Check sheet for the modelled part. Datum: model origin and axes. Units: mm. A direction names the side the tool comes from. Give positions to 0.01 mm unless a question says otherwise; leave off trailing zeros. Loops run counter-clockwise (first coordinate to the right, second up) from the corner with the lowest first, then second, coordinate; pieces in that order, holes last.
```python
from build123d import *

# Parameters (mm, degrees)
F0_W      = 127
F0_H      = 127
F1_DEPTH  = 7.62
F2_W      = 111.76
F2_H      = 7.62
F3_DEPTH  = 76.2
F4_W      = 25.4
F4_H      = 50.8
F5_DEPTH  = 7.62
F6_W      = 31.75
F6_H      = 19.05
F7_DEPTH  = 7.62
F8_W      = 38.1
F8_H      = 19.05
F9_DEPTH  = 7.62
F10_W     = 127
F10_H     = 127
F11_DEPTH = 7.62
F12_W     = 30.48
F12_H     = 38.1
F13_DEPTH = 7.62


with BuildPart() as f1:
    # F0 (on Top) → F1 (new body)
    with BuildSketch(Plane.XY):
        Rectangle(F0_W, F0_H)
    extrude(amount=F1_DEPTH)

    # F2 (on face) → F3 (join)
    with BuildSketch(Plane.XY.offset(7.62)):
        Polygon((-55.88, 63.5), (-63.5, 63.5), (-63.5, -63.5), (-55.88, -63.5), (-55.88, -55.88), (-55.88, 55.88), align=None)
        with Locations((0, 59.69)):
            Rectangle(F2_W, F2_H)
        Polygon((63.5, 63.5), (55.88, 63.5), (55.88, 55.88), (55.88, -55.88), (55.88, -63.5), (63.5, -63.5), align=None)
        with Locations((0, -59.69)):
            Rectangle(F2_W, F2_H)
    extrude(amount=F3_DEPTH)

    # F4 (on face) → F5 (cut, through all)
    with BuildSketch(Plane.YZ.offset(63.5)):
        with Locations((0, 33.02)):
            Rectangle(F4_W, F4_H)
    extrude(amount=-F5_DEPTH, mode=Mode.SUBTRACT)

    # F6 (on face) → F7 (cut, through all)
    with BuildSketch(Plane(origin=(0, 63.5, 0), x_dir=(-1, 0, 0), z_dir=(0, 1, 0))):
        with Locations((-32.296811, 61.150191)):
            Rectangle(F6_W, F6_H)
        with Locations((28.935332, 61.150191)):
            Rectangle(F6_W, F6_H)
    extrude(amount=-F7_DEPTH, mode=Mode.SUBTRACT)

    # F8 (on face) → F9 (cut, through all)
    with BuildSketch(Plane(origin=(-63.5, 0, 0), x_dir=(0, -1, 0), z_dir=(-1, 0, 0))):
        with Locations((-36.095939, 60.058468)):
            Rectangle(F8_W, F8_H)
        with Locations((35.046541, 60.058468)):
            Rectangle(F8_W, F8_H)
    extrude(amount=-F9_DEPTH, mode=Mode.SUBTRACT)

    # F10 (on face) → F11 (join)
    with BuildSketch(Plane.XY.offset(83.82)):
        Rectangle(F10_W, F10_H)
    extrude(amount=F11_DEPTH)

    # F12 (on face) → F13 (cut, through all)
    with BuildSketch(Plane.XZ.offset(63.5)):
        with Locations((-30.503813, 26.67)):
            Rectangle(F12_W, F12_H)
    extrude(amount=-F13_DEPTH, mode=Mode.SUBTRACT)


solid = f1.part
```
(1) Section check C-C on x = 3.5. Record the boundary of the cut face in (y, z).
(2) Access from +Z, -Z, +X, -X, +Y, -Y to the whole of each face (thin tool, end or side, straight path). Record for faces 5 (the face through (-29, 60, 51.625)), 6 (the face through (-60, -54.097, 60)), 7 (the face through (-63.5, -1, 45)), 8 (the face through (-1, -55.88, 45)).
(3) Section check B-B on z = 34.5. Record the boundary of the cut face in (x, y), plus the area to 3 significant figures.
(4) Section check D-D on z = 64.5. Record the boundary of the cut face in (x, y), plus the area to 3 significant figures.
(5) Release check for a two-part mould opening along Y. For faces 1 (the face through (60, 12.7, 33)), 2 (the face through (-60, 36, 50.533)), 3 (the face through (-1, 63.5, 45)), 4 (the face through (48.172, 60, 61)) record: pulls with the +Y half, pulls with the -Y half, needs draft (parallel to the pull), parting line crosses it, or undercut.
(6) Material ranges on line 1 (Z direction, x = -21, y = -36.5); line 2 (Y direction, x = -13, z = 69.5), recorded low to high.
(7) Section check A-A on x = -19. Record the boundary of the cut face in (y, z), plus the area to 3 significant figures.
Computed values:
1. outline: (-63.5, 0) - (63.5, 0) - (63.5, 91.44) - (-63.5, 91.44) - close; hole (-55.88, 7.62) - (55.88, 7.62) - (55.88, 83.82) - (-55.88, 83.82) - close
2. face 5: +Y
2. face 6: -X
2. face 7: +Z, -Z, -X, +Y, -Y
2. face 8: none
3. outline: (-63.5, -63.5) - (-45.74, -63.5) - (-45.74, -55.88) - (-55.88, -55.88) - (-55.88, 55.88) - (55.88, 55.88) - (55.88, 12.7) - (63.5, 12.7) - (63.5, 63.5) - (-63.5, 63.5) - close; (-15.26, -63.5) - (63.5, -63.5) - (63.5, -12.7) - (55.88, -12.7) - (55.88, -55.88) - (-15.26, -55.88) - close
3. area: 3,210 mm2
4. outline: (-63.5, -63.5) - (63.5, -63.5) - (63.5, 63.5) - (48.17, 63.5) - (48.17, 55.88) - (55.88, 55.88) - (55.88, -55.88) - (-55.88, -55.88) - (-55.88, -54.1) - (-63.5, -54.1) - close; (-63.5, -16) - (-55.88, -16) - (-55.88, 17.05) - (-63.5, 17.05) - close; (-63.5, 55.15) - (-55.88, 55.15) - (-55.88, 55.88) - (-44.81, 55.88) - (-44.81, 63.5) - (-63.5, 63.5) - close; (-13.06, 55.88) - (16.42, 55.88) - (16.42, 63.5) - (-13.06, 63.5) - close
4. area: 2,570 mm2
5. face 1: undercut
5. face 2: undercut
5. face 3: pulls with the +Y half
5. face 4: needs draft
6. line 1: z = 0 to 7.62, 83.82 to 91.44
6. line 2: y = -63.5 to -55.88, 55.88 to 63.5
7. outline: (-63.5, 0) - (63.5, 0) - (63.5, 51.63) - (55.88, 51.63) - (55.88, 7.62) - (-63.5, 7.62) - close; (-63.5, 45.72) - (-55.88, 45.72) - (-55.88, 83.82) - (55.88, 83.82) - (55.88, 70.68) - (63.5, 70.68) - (63.5, 91.44) - (-63.5, 91.44) - close
7. area: 2,660 mm2
